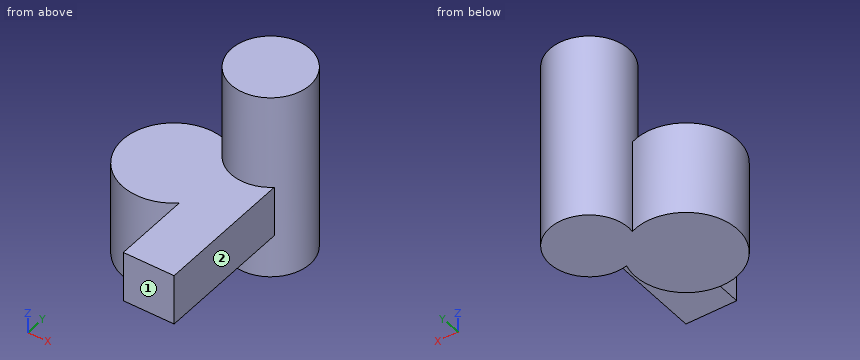
from build123d import *

# Parameters (mm, degrees)
F1_R     = 4.2
F2_R     = 5.45
F7_W     = 5.4
F7_H     = 19.2
F8_DEPTH = 5.4


with BuildPart() as f5:
    # F5: sweep along a path in F4
    with BuildLine(Plane(origin=(0, 0, 0), x_dir=(0.744048, 0.668127, 0), z_dir=(0.668127, -0.744048, 0))) as f5_path:
        Line((0, 0), (0, 20))
    # F1 (on Top) → F5 (sweep)
    with BuildSketch(Plane.XY):
        Circle(F1_R)
    sweep(path=f5_path.line)

    # F6: sweep along a path in F4
    with BuildLine(Plane(origin=(0, 0, 0), x_dir=(0.744048, 0.668127, 0), z_dir=(0.668127, -0.744048, 0))) as f6_path:
        Line((-8.4, 0), (-8.4, 10))
    # F2 (on Top) → F6 (sweep)
    with BuildSketch(Plane.XY):
        with Locations((-6.25, -5.612263)):
            Circle(F2_R)
    sweep(path=f6_path.line)

    # F7 (on face) → F8 (join)
    with BuildSketch(Plane.XY.offset(10)):
        with Locations((0, -8.4)):
            Rectangle(F7_W, F7_H)
    extrude(amount=-F8_DEPTH)


solid = f5.part
The listing builds one solid part. Answer for the finished solid, in the listing's coordinates (mm). Face numbers are marked on the shaded views. A direction names the side the tool comes from. Coordinates: 2 decimals unless noted, no trailing zeros. Write each loop counter-clockwise with the first axis right and the second up, starting at its lowest first coordinate (ties: lowest second). Pieces come first, ordered by that corner, then holes. Notation, with made-up numbers: (30.5, 62.25) - (46.5, 62.25) arc R23 ccw to (46.5, 86.25) - close; hole circle Ø8 at (79, 2.5). An arc over 180 degrees is marked (long way). Return JSON: item names as keys, results as strings.
1. The part is cut by section A-A on x = 0. Determine the outline of the cut face in (y, z), then the cut area to 3 significant figures.
Final values:
{"outline": "(-18, 4.6) - (-4.2, 4.6) - (-4.2, 0) - (4.2, 0) - (4.2, 20) - (-4.2, 20) - (-4.2, 10) - (-18, 10) - close", "area": "243 mm^2"}
2. The part is cut by section B-B on y = -13.25. Determine the outline of the cut face in (x, z), then the cut area to 3 significant figures.
Final values:
{"outline": "(-2.7, 4.6) - (2.7, 4.6) - (2.7, 10) - (-2.7, 10) - close", "area": "29.2 mm^2"}
3. Consider line 1 along Z through (x, y) = (-3.25, -10); line 2 along Y through (x, z) = (-6, 2.75); line 3 along Z through (x, y) = (0, -7.25). Determine where each line is inside the solid, lowest interval first.
Final values:
{"line 1": "0 to 10", "line 2": "-11.06 to -0.17", "line 3": "4.6 to 10"}
4. Which of the six approach directions +Z, -Z, +X, -X, +Y, -Y give full straight-line access (tool end or side, diameter ignored) to the marked faces 1 and 2?
Final values:
{"face 1": "+Z, -Z, +X, -X, -Y", "face 2": "+Z, -Z, +X, -Y"}
5. Each of these flat-tipped pins is pushed along its axis until it touches: pin 1 Ø2 at (y, z) = (-7, 15) entering from +X; pin 2 Ø1.5 at (x, y) = (-5.5, -11) entering from +Z; pin 3 Ø2 at (x, y) = (-8, -6) entering from -Z; pin 4 Ø2 at (y, z) = (0, 17.5) entering from -X. Where does it stop, or does it pass through?
Final values:
{"pin 1": "through", "pin 2": "z = 10", "pin 3": "z = 0", "pin 4": "x = -4.2"}
6. The part is cut by section D-D on y = -3.5. Determine the outline of the cut face in (x, z).
Final values:
{"outline": "(-11.27, 0) - (2.32, 0) - (2.32, 4.6) - (2.7, 4.6) - (2.7, 10) - (2.32, 10) - (2.32, 20) - (-2.32, 20) - (-2.32, 10) - (-11.27, 10) - close"}
7. The part is cut by section C-C on z = 8.5. Determine the outline of the cut face in (x, y), then the cut area to 3 significant figures.
Final values:
{"outline": "(-4.16, -0.58) arc R5.45 ccw (long way) to (-2.7, -9.75) - (-2.7, -18) - (2.7, -18) - (2.7, -3.22) arc R4.2 ccw (long way) to start", "area": "212 mm^2"}
